Geometry check sheet. Reference: the model listing, model coordinates, mm. Face numbers are marked on the shaded views. A direction names the side the tool comes from. Coordinates: 2 decimals unless noted, no trailing zeros. Loops run counter-clockwise (first coordinate to the right, second up) from the corner with the lowest first, then second, coordinate; pieces in that order, holes last.
from build123d import *

# Parameters (mm, degrees)
F0_W     = 150.370433
F0_H     = 150.421701
F1_DEPTH = 65.024
F2_T     = -2.54


with BuildPart() as f1:
    # F0 (on Top) → F1 (new body)
    with BuildSketch(Plane.XY):
        with Locations((0.977538, 0.564386)):
            Rectangle(F0_W, F0_H)
    extrude(amount=-F1_DEPTH)

    # F2
    f2_openings = [f1.faces().sort_by_distance(p)[0] for p in [
        (0.977539, 0.564385, -65.024),
    ]]
    offset(amount=F2_T, openings=f2_openings)


solid = f1.part
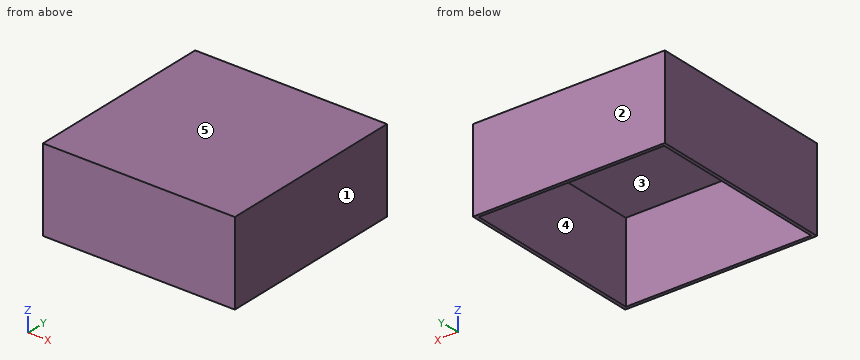
(1) Gauge pin test, flat end, axial feed: pin 1 Ø3 at (x, y) = (-36, -11) entering from -Z. Record the tip position at first contact, or that the pin passes through.
Findings:
pin 1: stops at z = -2.54
(2) Scan lines: L1, parallel to Y at x = 18, z = -23; L2, parallel to X at y = -15, z = -10; L3, parallel to Z at x = -2.5, y = -55. Record each from-to range of solid material in increasing order.
Findings:
L1: y = -74.65 to -72.11, 73.24 to 75.78
L2: x = -74.21 to -71.67, 73.62 to 76.16
L3: z = -2.54 to 0
(3) Sectioned sample at A-A on z = -27. Record the cut outline in (x, y), and give its area (3 significant figures).
Findings:
outline: (-74.21, -74.65) - (76.16, -74.65) - (76.16, 75.78) - (-74.21, 75.78) - close; hole (-71.67, -72.11) - (73.62, -72.11) - (73.62, 73.24) - (-71.67, 73.24) - close
area: 1,500 mm2
(4) Draft check along X on the marked faces 1, 2 and 3. Enter one of: +X half, -X half, draft (parallel to the pull), parting line (faces both ways), or undercut.
Findings:
face 1: +X half
face 2: draft
face 3: undercut
(5) Access from +Z, -Z, +X, -X, +Y, -Y to the whole of each face (thin tool, end or side, straight path). Record for the marked faces 4 and 5.
Findings:
face 4: -Z
face 5: +Z, +X, -X, +Y, -Y
(6) Sectioned sample at C-C on y = -42.5. Record the cut outline in (x, z).
Findings:
outline: (-74.21, -65.02) - (-71.67, -65.02) - (-71.67, -2.54) - (73.62, -2.54) - (73.62, -65.02) - (76.16, -65.02) - (76.16, 0) - (-74.21, 0) - close
(7) Sectioned sample at B-B on x = -25.5. Record the cut outline in (y, z).
Findings:
outline: (-74.65, -65.02) - (-72.11, -65.02) - (-72.11, -2.54) - (73.24, -2.54) - (73.24, -65.02) - (75.78, -65.02) - (75.78, 0) - (-74.65, 0) - close
